Model file for the job. Use its own axes, mm. Face numbers are marked on the shaded views. A direction names the side the tool comes from. Round coordinates to 2 decimals unless told otherwise and drop trailing zeros. Order: outer loops, then holes, each group sorted by start corner. A loop starts at its lowest first (then second) coordinate and runs counter-clockwise, first axis right, second up. Notation, with made-up numbers: (73.5, 33) -> (121.5, 33) arc R25 cw to (121.5, 47) -> close; hole circle Ø8 at (61.5, 38). An arc over 180 degrees is marked (long way). Answer as CSV lines item,"result".
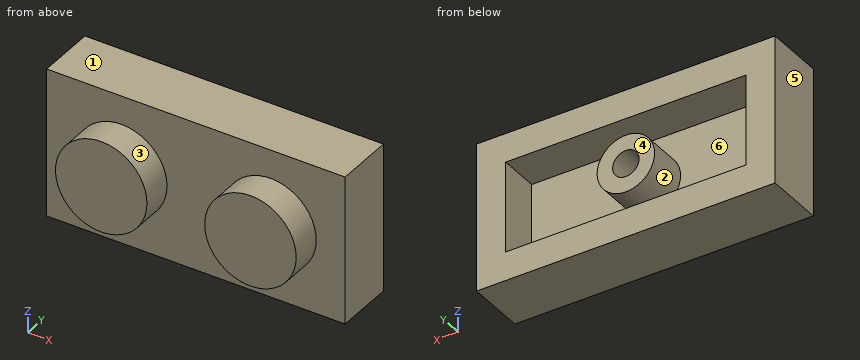
```python
from build123d import *

# Parameters (mm, degrees)
F0_R     = 2.44
F1_DEPTH = 3.15
F2_DEPTH = 4.8
F3_W     = 12.82
F3_H     = 4.85
F3_R     = 1.53
F3_R_2   = 0.705
F4_DEPTH = 2.14


with BuildPart() as f1:
    # F0 (on Front) → F1 (new body)
    with BuildSketch(Plane.XZ):
        Polygon((2.131469, 8.320145), (-13.788531, 8.320145), (-13.788531, 0.390145), (-10.388192, 0.390145), (-7.928192, 0.390145), (-3.748192, 0.390145), (-1.288192, 0.390145), (2.131469, 0.390145), align=None)
        with Locations((-9.808531, 4.355145)):
            Circle(F0_R, mode=Mode.SUBTRACT)
        with Locations((-1.848531, 4.355145)):
            Circle(F0_R, mode=Mode.SUBTRACT)
    extrude(amount=F1_DEPTH)

    # F0 (on Front) → F2 (join)
    with BuildSketch(Plane.XZ):
        with Locations((-9.808531, 4.355145)):
            Circle(F0_R)
        with Locations((-1.848531, 4.355145)):
            Circle(F0_R)
    extrude(amount=F2_DEPTH)

    # F3 (on face) → F4 (cut)
    with BuildSketch(Plane(origin=(0, 0, 0), x_dir=(-1, 0, 0), z_dir=(0, 1, 0))):
        with Locations((5.828531, 4.355145)):
            Rectangle(F3_W, F3_H)
        with Locations((5.828531, 4.355145)):
            Circle(F3_R, mode=Mode.SUBTRACT)
        with Locations((5.828531, 4.355145)):
            Circle(F3_R_2)
    extrude(amount=-F4_DEPTH, mode=Mode.SUBTRACT)


solid = f1.part
```
Q1. Saw through at C-C (x = -11.25). Write the cut outline in (y, z), plus the area to 3 significant figures.
Checks:
outline,"(-4.8, 2.39) -> (-3.15, 2.39) -> (-3.15, 0.39) -> (0, 0.39) -> (0, 1.93) -> (-2.14, 1.93) -> (-2.14, 6.78) -> (0, 6.78) -> (0, 8.32) -> (-3.15, 8.32) -> (-3.15, 6.32) -> (-4.8, 6.32) -> close"
area,"21.1 mm²"
Q2. Saw through at A-A (y = -0.6). Write the cut outline in (x, z) (3 decimals), plus the area to 3 significant figures.
Checks:
outline,"(-13.789, 0.39) -> (2.131, 0.39) -> (2.131, 8.32) -> (-13.789, 8.32) -> close; circle Ø3.06 at (-5.829, 4.355); hole (-12.239, 1.93) -> (0.581, 1.93) -> (0.581, 6.78) -> (-12.239, 6.78) -> close; hole circle Ø1.41 at (-5.829, 4.355)"
area,"69.9 mm²"
Q3. Wall check: L1, parallel to X at y = -0.7, z = 6.75; L2, parallel to Z at x = -6, y = -1.9; L3, parallel to Z at x = -4.25, y = -1.9. Give the ranges that are in metal, low to high. Write a range as [from, to].
Checks:
L1,"[-13.79, -12.24], [0.58, 2.13]"
L2,"[0.39, 1.93], [2.83, 3.67], [5.04, 5.88], [6.78, 8.32]"
L3,"[0.39, 1.93], [6.78, 8.32]"
Q4. Saw through at B-B (z = 4). Write the cut outline in (x, y), plus the area to 3 significant figures.
Checks:
outline,"(-13.79, -3.15) -> (-12.22, -3.15) -> (-12.22, -4.8) -> (-7.39, -4.8) -> (-7.39, -3.15) -> (-4.26, -3.15) -> (-4.26, -4.8) -> (0.57, -4.8) -> (0.57, -3.15) -> (2.13, -3.15) -> (2.13, 0) -> (0.58, 0) -> (0.58, -2.14) -> (-4.34, -2.14) -> (-4.34, 0) -> (-5.22, 0) -> (-5.22, -2.14) -> (-6.44, -2.14) -> (-6.44, 0) -> (-7.32, 0) -> (-7.32, -2.14) -> (-12.24, -2.14) -> (-12.24, 0) -> (-13.79, 0) -> close"
area,"42.4 mm²"
Q5. Mould opens along X. For the marked faces 4, 5 and 6 say: +X half, -X half, draft (parallel to the pull), parting line (faces both ways), or undercut.
Checks:
face 4,"draft"
face 5,"-X half"
face 6,"undercut"
Q6. Tool access for the marked faces 1, 2 and 3: list every direction of +Z, -Z, +X, -X, +Y, -Y with a clear straight run to the whole face (end or side of a thin tool).
Checks:
face 1,"+Z, +X, -X, +Y, -Y"
face 2,"+Y"
face 3,"-Y"
Q7. Flat gauge pins, fed straight in: pin 1 (3 mm diameter, centred on x = -8.5, z = 5.5, fed in from +Y); pin 2 (1.8 mm diameter, centred on x = -5.83, z = 4.36, fed in from -Y). Where does each tip first touch, or does it go through?
Checks:
pin 1,"y = 0"
pin 2,"y = -3.15"
Q8. Saw through at D-D (y = -3.7). Write the cut outline in (x, z).
Checks:
outline,"circle Ø4.88 at (-9.81, 4.36); circle Ø4.88 at (-1.85, 4.36)"
